The model under review builds one solid part; all positions refer to its coordinate system, in mm. Face numbers are marked on the shaded views. A direction names the side the tool comes from. Give positions to 0.01 mm unless a question says otherwise; leave off trailing zeros. Loops run counter-clockwise (first coordinate to the right, second up) from the corner with the lowest first, then second, coordinate; pieces in that order, holes last. Notation, with made-up numbers: M 18,-39 L 75,-39 A16 cw 75,-14 Z; hole C 3,89.5 d2. An arc over 180 degrees is marked long. Write item = value, one per line. Start each with the question number.
1. We need section B-B on x = 0. Give the boundary of the cut face in (y, z), then the cut area to 3 significant figures.
2. For pin 1 (8 mm diameter, centred on y = 18.5, z = 80.5, fed in from +X); pin 2 (12 mm diameter, centred on y = 9.5, z = 17.5, fed in from -X); pin 3 (3 mm diameter, centred on y = 22.5, z = 79.5, fed in from -X); pin 4 (8 mm diameter, centred on y = -4.5, z = -41, fed in from +X), all flat-tipped, find the tip position at first contact; note any pin that passes through.
3. We need section A-A on y = 20.5. Give the boundary of the cut face in (x, z), then the cut area to 3 significant figures.
4. For the marked faces 1 and 2, list the 3-axis set-ups (+Z, -Z, +X, -X, +Y, -Y) from which the entire face can be reached by the end or side of a thin tool; tool diameter is ignored.
5. Draft analysis for pull direction Z (two halves, no side actions). For the marked faces 3, 4 and 5, state which applies: pulls with the +Z half, pulls with the -Z half, needs draft (parallel to the pull), parting line crosses it, or undercut.
6. We need section C-C on z = -42. Give the boundary of the cut face in (x, y), then the cut area to 3 significant figures.
7. Wall thickness on line 1 along Z through (x, y) = (45, 16); line 2 along Z through (x, y) = (48, 19); line 3 along Y through (x, z) = (-79.5, 33): over which ranges is each line inside the solid? List them lowest first. Write a range as from..to.
8. We need section D-D on x = 34. Give the boundary of the cut face in (y, z).
from build123d import *

# Parameters (mm, degrees)
SKETCH1_R           = 127
BOSS_EXTRUDE1_DEPTH = 25.4
CUT_EXTRUDE1_DEPTH  = 10.16
SKETCH3_R           = 12.7
BOSS_EXTRUDE2_DEPTH = 38.1


with BuildPart() as part:
    # Sketch1 → Boss-Extrude1 (new body)
    with BuildSketch(Plane(origin=(0, 0, 0), x_dir=(1, 0, 0), z_dir=(0, 1, 0))):
        with Locations(Location((0, 0, 0), (0, 0, 270))):
            Circle(SKETCH1_R)
    extrude(amount=BOSS_EXTRUDE1_DEPTH)

    # Sketch2 → Cut-Extrude1 (cut)
    with BuildSketch(Plane(origin=(0, 25.4, 0), x_dir=(1, 0, 0), z_dir=(0, 1, 0))):
        Polygon((12.7, -127), (12.7, -21.997045256), (103.635226281, -74.498522628), (138.332271537, -74.498522628), (116.335226281, -52.501477372), (25.4, 0), (116.335226281, 52.501477372), (130.311019476, 77.4940315), (103.635226281, 74.498522628), (12.7, 21.997045256), (12.7, 127), (0, 157.984531472), (-12.7, 127), (-12.7, 21.997045256), (-103.635226281, 74.498522628), (-124.892355956, 78.379341128), (-116.335226281, 52.501477372), (-25.4, 0), (-116.335226281, -52.501477372), (-133.449485631, -77.846459753), (-103.635226281, -74.498522628), (-12.7, -21.997045256), (-12.7, -127), (12.7, -156.136703653), align=None)
    extrude(amount=-CUT_EXTRUDE1_DEPTH, mode=Mode.SUBTRACT)

    # Sketch3 → Boss-Extrude2 (add)
    with BuildSketch(Plane(origin=(0, 0, 0), x_dir=(-1, 0, 0), z_dir=(0, -1, 0))):
        with Locations(Location((0, 0, 0), (0, 0, 270))):
            Circle(SKETCH3_R)
    extrude(amount=BOSS_EXTRUDE2_DEPTH)


solid = part.part
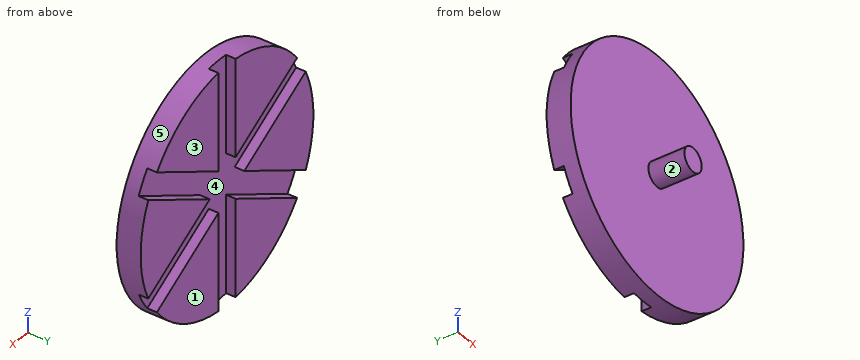
Final values:
q1.outline = M -38.1,-12.7 L 0,-12.7 L 0,-127 L 15.24,-127 L 15.24,127 L 0,127 L 0,12.7 L -38.1,12.7 Z
q1.area = 4,840 mm²
q2.pin_1 = 101.37
q2.pin_2 = -126.48
q2.pin_3 = -100.22
q2.pin_4 = through
q3.outline = M -115.78,-52.18 L -25.4,0 L -115.78,52.18 A127 ccw Z; M -103.08,-74.18 A127 ccw -12.7,-126.36 L -12.7,-22 Z; M -103.08,74.18 L -12.7,22 L -12.7,126.36 A127 ccw Z; M 12.7,-126.36 A127 ccw 103.08,-74.18 L 12.7,-22 Z; M 12.7,22 L 103.08,74.18 A127 ccw 12.7,126.36 Z; M 25.4,0 L 115.78,-52.18 A127 ccw 115.78,52.18 Z
q3.area = 33,000 mm²
q4.face_1 = +Z, -Z, +X, -X, +Y
q4.face_2 = -Y
q5.face_3 = needs draft
q5.face_4 = undercut
q5.face_5 = parting line crosses it
q6.outline = M -119.85,0 L 119.85,0 L 119.85,25.4 L 98.15,25.4 L 98.15,15.24 L 47.35,15.24 L 47.35,25.4 L 12.7,25.4 L 12.7,15.24 L -12.7,15.24 L -12.7,25.4 L -47.35,25.4 L -47.35,15.24 L -98.15,15.24 L -98.15,25.4 L -119.85,25.4 Z
q6.area = 4,800 mm²
q7.line_1 = -118.76..-40.65, -11.32..11.32, 40.65..118.76
q7.line_2 = -117.58..-42.38, -13.05..13.05, 42.38..117.58
q7.line_3 = 0..15.24
q8.outline = M 0,-122.36 L 25.4,-122.36 L 25.4,-34.29 L 15.24,-34.29 L 15.24,-4.97 L 25.4,-4.97 L 25.4,4.97 L 15.24,4.97 L 15.24,34.29 L 25.4,34.29 L 25.4,122.36 L 0,122.36 Z
